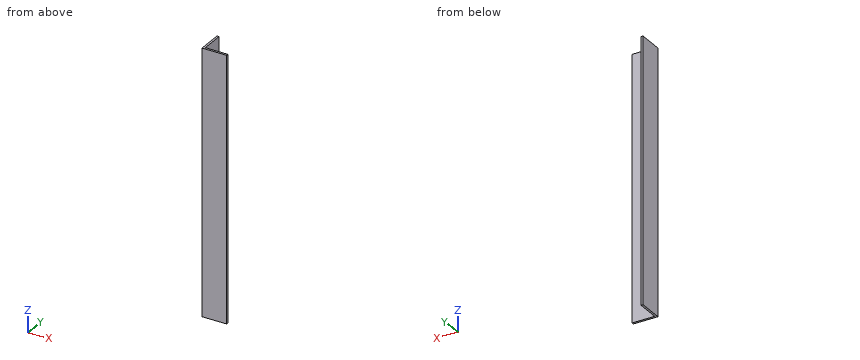
Autodesk Inventor part; units mm, degrees
ref_plane "YZ Plane" through (0, 0, 0) normal (1, 0, 0) x (0, 1, 0)
ref_plane "XZ Plane" through (0, 0, 0) normal (0, 1, 0) x (-1, 0, 0)
ref_plane "XY Plane" through (0, 0, 0) normal (0, 0, 1) x (1, 0, 0)
sketch "Sketch1" plane through (0, 0, 0) normal (0, 0, 1) x (1, 0, 0)
  line L0 (0, 0) -> (38.1, 0)
  line L1 (38.1, 0) -> (38.1, 3.175)
  line L2 (38.1, 3.175) -> (0, 3.175)
  line L3 (0, 3.175) -> (0, 0)
  dimension "d0" = 38.1
  dimension "d1" = 3.175
extrude "Extrusion1" add sketch "Sketch1" along normal blind 355.6
sketch "Sketch2" plane through (0, 0, 355.6) normal (0, 0, 1) x (1, 0, 0)
  line L0 (0, 0) -> (3.175, 0)
  line L1 (3.175, 0) -> (3.175, 38.1)
  line L2 (3.175, 38.1) -> (0, 38.1)
  line L3 (0, 38.1) -> (0, 0)
  dimension "d4" = 3.175
  dimension "d5" = 38.1
extrude "Extrusion2" add sketch "Sketch2" against normal blind 355.6
sketch "Sketch3" plane through (0, 0, 355.6) normal (0, 0, 1) x (1, 0, 0)
  line L0 (0, 0) -> (38.1, 0)
  line L1 (38.1, 0) -> (38.1, 3.175)
  line L2 (38.1, 3.175) -> (3.175, 3.175)
  line L3 (38.1, 3.175) -> (3.175, 3.175)
  line L4 (3.175, 3.175) -> (3.175, 38.1)
  line L5 (3.175, 38.1) -> (0, 38.1)
  line L6 (0, 38.1) -> (0, 0)
  line L7 (0, 38.1) -> (0, 0)
extrude "Extrusion3" add sketch "Sketch3" along normal blind 50.8
properties part number "16in 2inL"
Source: CAD feature listing. Evaluate the final solid. Frame: model axes, mm. Give positions to 0.01 mm unless a question says otherwise; leave off trailing zeros. Order: outer loops, then holes, each group sorted by start corner. A loop starts at its lowest first (then second) coordinate and runs counter-clockwise, first axis right, second up. Notation, with made-up numbers: (78, -33.5) -> (124, -33.5) arc R17 ccw to (124, -3.5) -> close; hole circle Ø1 at (30, 52). An arc over 180 degrees is marked (long way). Use a Markdown table: item, result.
1) Ray query, line 1 along Y through (x, z) = (18, 343) (3 decimals). Return the intervals inside material, ascending. Write a range as [from, to].
Answer list:
| item | result |
|---|---|
| line 1 | [0, 3.175] |
2) Contact query for flat-ended pins moving along their axis: P1, Ø6, axis at y = 4.5, z = 141.5, coming from the +X side; P2, Ø3, axis at x = 13, y = 5, coming from the +Z side; P3, Ø5, axis at y = 21.5, z = 340, coming from the +X side (3 decimals). Output: stop coordinate, or through.
Answer list:
| item | result |
|---|---|
| P1 | x = 38.1 |
| P2 | through |
| P3 | x = 3.175 |
3) Section query A-A, the plane z = 64.5. Return the cut outline in (x, y) (3 decimals), then the cut area to 3 significant figures.
Answer list:
| item | result |
|---|---|
| outline | (0, 0) -> (38.1, 0) -> (38.1, 3.175) -> (3.175, 3.175) -> (3.175, 38.1) -> (0, 38.1) -> close |
| area | 232 mm² |
4) Section query B-B, the plane y = 9.5. Return the cut outline in (x, z) (3 decimals), then the cut area to 3 significant figures.
Answer list:
| item | result |
|---|---|
| outline | (0, 0) -> (3.175, 0) -> (3.175, 406.4) -> (0, 406.4) -> close |
| area | 1,290 mm² |
